Input: dimensioned drawing with shaded views. Units: mm. Origin: part minimum x, y, z. A direction names the side the tool comes from. Round coordinates to 2 decimals unless told otherwise and drop trailing zeros. Order: outer loops, then holes, each group sorted by start corner. A loop starts at its lowest first (then second) coordinate and runs counter-clockwise, first axis right, second up.
Item 1: Line query: L1, parallel to Z at x = 6.75, y = 6.75; L2, parallel to Y at x = 10.75, z = 23; L3, parallel to Z at x = 3.5, y = 7. Output: solid intervals per line, ascending.
Item 2: Cut plane B-B on y = 6.75. Output: boundary loops of the cut face in (x, z), then the cut area to 3 significant figures.
Item 3: Cut plane A-A on z = 8.5. Output: boundary loops of the cut face in (x, y), then the cut area to 3 significant figures.
Item 4: First-contact query: pin 1 (1.5 mm diameter, centred on y = 7, z = 23, fed in from -X); pin 2 (6 mm diameter, centred on x = 3, z = 32, fed in from -Y); pin 3 (0.9 mm diameter, centred on y = 6.5, z = 19, fed in from +X); pin 4 (6 mm diameter, centred on x = 13, z = 31.5, fed in from +Y). Flat tips, straight axial feed; report the tip coordinate or a pass-through.
Item 5: Cut plane C-C on z = 26. Output: boundary loops of the cut face in (x, y).
Item 6: Cut plane D-D on x = 6.5. Give the number of separate pieces and of enclosed holes in the cut face, then the cut area to 3 significant figures.
Item 7: Reachability of the marked faces 1 and 2 from +Z, -Z, +X, -X, +Y, -Y: full face, straight path, thin tool, end or side. Return the list, or none.
Item 8: Mould query, pull axis Z, two halves, no side actions, for the marked faces 3, 4 and 5. Classes: released by +Z, released by -Z, zero draft, split by the parting line, or undercut.
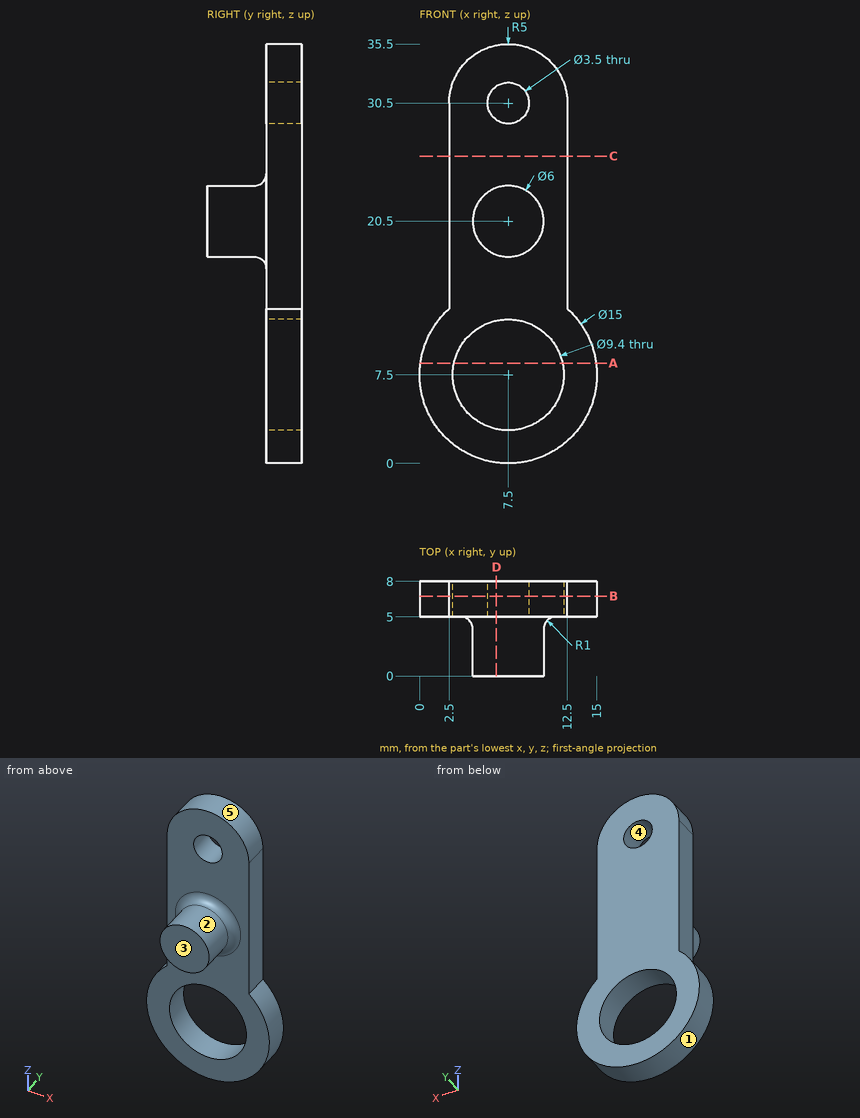
From the geometry:
1. L1: z = 0.04 to 2.86, 12.14 to 28.92, 32.08 to 35.44
1. L2: y = 5 to 8
1. L3: z = 1.16 to 5.03, 9.97 to 33.5
2. outline: (2.5, 13.09) arc R7.5 ccw (long way) to (12.5, 13.09) - (12.5, 30.5) arc R5 ccw to (2.5, 30.5) - close; hole circle Ø9.4 at (7.5, 7.5); hole circle Ø3.5 at (7.5, 30.5)
2. area: 298 mm2
3. outline: (0.07, 5) - (2.91, 5) - (2.91, 8) - (0.07, 8) - close; (12.09, 5) - (14.93, 5) - (14.93, 8) - (12.09, 8) - close
3. area: 17.0 mm2
4. pin 1: stops at x = 2.5
4. pin 2: stops at y = 5
4. pin 3: stops at x = 12.5
4. pin 4: stops at y = 8
5. outline: (2.5, 5) - (12.5, 5) - (12.5, 8) - (2.5, 8) - close
6. separate pieces: 3
6. enclosed holes: 0
6. area: 98.6 mm2
7. face 1: +Y, -Y
7. face 2: -Y
8. face 3: zero draft
8. face 4: undercut
8. face 5: released by +Z
